from build123d import *

# Parameters (mm, degrees)
SKETCH1_W                     = 20
SKETCH1_H                     = 365
BOSS_EXTRUDE1_DEPTH           = 1.5875
CSK_FOR_M4_SFHCS1_AT_2_COUNT  = 2
CSK_FOR_M4_SFHCS1_AT_2_PITCH  = 14.142135624
CSK_FOR_M4_SFHCS1_AT_3_COUNT  = 2
CSK_FOR_M4_SFHCS1_AT_3_PITCH  = 10
CSK_FOR_M4_SFHCS1_AT_4_COUNT  = 2
CSK_FOR_M4_SFHCS1_AT_4_PITCH  = 10
CSK_FOR_M4_SFHCS1_AT_5_COUNT  = 2
CSK_FOR_M4_SFHCS1_AT_5_PITCH  = 346
CSK_FOR_M4_SFHCS1_AT_6_COUNT  = 2
CSK_FOR_M4_SFHCS1_AT_6_PITCH  = 336.148776586
CSK_FOR_M4_SFHCS1_AT_7_COUNT  = 2
CSK_FOR_M4_SFHCS1_AT_7_PITCH  = 346.144478506
CSK_FOR_M4_SFHCS1_AT_8_COUNT  = 2
CSK_FOR_M4_SFHCS1_AT_8_PITCH  = 336
CSK_FOR_M4_SFHCS1_AT_9_COUNT  = 2
CSK_FOR_M4_SFHCS1_AT_9_PITCH  = 260
CSK_FOR_M4_SFHCS1_AT_10_COUNT = 2
CSK_FOR_M4_SFHCS1_AT_10_PITCH = 290
M4X0_7_TAPPED_HOLE1_D         = 3.3


with BuildPart() as part:
    # Sketch1 → Boss-Extrude1 (new body)
    with BuildSketch(Plane(origin=(0, 0, 0), x_dir=(1, 0, 0), z_dir=(0, 1, 0))):
        Rectangle(SKETCH1_W, SKETCH1_H)
    extrude(amount=BOSS_EXTRUDE1_DEPTH)

    # Sketch3 → CSK for M4 SFHCS1 (revolve, cut)
    with BuildSketch(Plane(origin=(5, 1.5875, 168), x_dir=(0, 0, 1), z_dir=(1, 0, 0))):
        Polygon((0, 0), (0, 1.5875), (2.25, 1.5875), (2.25, 2.23), (4.48, 0), align=None)
    csk_for_m4_sfhcs1 = revolve(axis=Axis((5, 7.9375, 168), (0, -1, 0)), mode=Mode.SUBTRACT)

    # CSK for M4 SFHCS1 at 2: CSK for M4 SFHCS1 ×2
    with Locations(*[Vector(-0.7071067811865469, 0, 0.7071067811865482) * (i * CSK_FOR_M4_SFHCS1_AT_2_PITCH) for i in range(1, CSK_FOR_M4_SFHCS1_AT_2_COUNT)]):
        add(csk_for_m4_sfhcs1, mode=Mode.SUBTRACT)

    # CSK for M4 SFHCS1 at 3: CSK for M4 SFHCS1 ×2
    with Locations(*[(-i * CSK_FOR_M4_SFHCS1_AT_3_PITCH, 0, 0) for i in range(1, CSK_FOR_M4_SFHCS1_AT_3_COUNT)]):
        add(csk_for_m4_sfhcs1, mode=Mode.SUBTRACT)

    # CSK for M4 SFHCS1 at 4: CSK for M4 SFHCS1 ×2
    with Locations(*[(0, 0, i * CSK_FOR_M4_SFHCS1_AT_4_PITCH) for i in range(1, CSK_FOR_M4_SFHCS1_AT_4_COUNT)]):
        add(csk_for_m4_sfhcs1, mode=Mode.SUBTRACT)

    # CSK for M4 SFHCS1 at 5: CSK for M4 SFHCS1 ×2
    with Locations(*[(0, 0, -i * CSK_FOR_M4_SFHCS1_AT_5_PITCH) for i in range(1, CSK_FOR_M4_SFHCS1_AT_5_COUNT)]):
        add(csk_for_m4_sfhcs1, mode=Mode.SUBTRACT)

    # CSK for M4 SFHCS1 at 6: CSK for M4 SFHCS1 ×2
    with Locations(*[Vector(-0.029748732396333223, 0, -0.9995574085167952) * (i * CSK_FOR_M4_SFHCS1_AT_6_PITCH) for i in range(1, CSK_FOR_M4_SFHCS1_AT_6_COUNT)]):
        add(csk_for_m4_sfhcs1, mode=Mode.SUBTRACT)

    # CSK for M4 SFHCS1 at 7: CSK for M4 SFHCS1 ×2
    with Locations(*[Vector(-0.028889670703889703, 0, -0.9995826063545828) * (i * CSK_FOR_M4_SFHCS1_AT_7_PITCH) for i in range(1, CSK_FOR_M4_SFHCS1_AT_7_COUNT)]):
        add(csk_for_m4_sfhcs1, mode=Mode.SUBTRACT)

    # CSK for M4 SFHCS1 at 8: CSK for M4 SFHCS1 ×2
    with Locations(*[(0, 0, -i * CSK_FOR_M4_SFHCS1_AT_8_PITCH) for i in range(1, CSK_FOR_M4_SFHCS1_AT_8_COUNT)]):
        add(csk_for_m4_sfhcs1, mode=Mode.SUBTRACT)

    # CSK for M4 SFHCS1 at 9: CSK for M4 SFHCS1 ×2
    with Locations(*[(0, 0, -i * CSK_FOR_M4_SFHCS1_AT_9_PITCH) for i in range(1, CSK_FOR_M4_SFHCS1_AT_9_COUNT)]):
        add(csk_for_m4_sfhcs1, mode=Mode.SUBTRACT)

    # CSK for M4 SFHCS1 at 10: CSK for M4 SFHCS1 ×2
    with Locations(*[(0, 0, -i * CSK_FOR_M4_SFHCS1_AT_10_PITCH) for i in range(1, CSK_FOR_M4_SFHCS1_AT_10_COUNT)]):
        add(csk_for_m4_sfhcs1, mode=Mode.SUBTRACT)

    # M4x0.7 Tapped Hole1 (through all)
    with Locations(Plane(origin=(0, 1.5875, 0), x_dir=(1, 0, 0), z_dir=(0, 1, 0))):
        with Locations((-5, -100), (-5, 100), (5, -100), (5, 0), (5, 102), (5, 112)):
            Hole(M4X0_7_TAPPED_HOLE1_D / 2)


solid = part.part
Read the model definition and answer for the solid it produces. Units are mm, in the model's axes. Round coordinates to 2 decimals unless told otherwise and drop trailing zeros.
1) The part is cut by section A-A on y = 1.25. Give the number of separate pieces and of enclosed holes in the cut face, plus the area to 3 significant figures.
2) A flat-ended cylindrical pin translates along its axis: pin 1 (12 mm diameter, centred on x = -1, z = 15.5, fed in from -Y). Find the tip coordinate at first contact, or state that the pin passes through.
3) Straight lines are drawn through the part: L1, parallel to X at y = 0.3, z = 100; L2, parallel to X at y = 0.4, z = -112; L3, parallel to Z at x = -2.25, y = 0.6. For each, find the intervals that lie inside material, in ascending order.
Resolved:
1. separate pieces: 1
1. enclosed holes: 16
1. area: 6,710 mm2
2. pin 1: stops at y = 0
3. L1: x = -10 to -6.65, -3.35 to 3.35, 6.65 to 10
3. L2: x = -10 to 3.35, 6.65 to 10
3. L3: z = -182.5 to -180.15, -175.85 to -170.15, -165.85 to 165.85, 170.15 to 175.85, 180.15 to 182.5
